Source: CAD feature listing. Evaluate the final solid. Frame: model axes, mm. A direction names the side the tool comes from. Give positions to 0.01 mm unless a question says otherwise; leave off trailing zeros. Write each loop counter-clockwise with the first axis right and the second up, starting at its lowest first coordinate (ties: lowest second). Pieces come first, ordered by that corner, then holes. Notation, with made-up numbers: (39, -34) -> (62, -34) arc R13 cw to (62, -10) -> close; hole circle Ø6 at (87, 86.5). An arc over 180 degrees is marked (long way). Write item = value, one per line.
from build123d import *

# Parameters (mm, degrees)
PAD_DEPTH   = 4
FILLET_R    = 25
SKETCH002_R = 1.25
HOLE_DEPTH  = 3
HOLE_TIPS_R = 1.25


with BuildPart() as part:
    # Sketch → Revolution (revolve)
    with BuildSketch(Plane.XZ):
        with BuildLine():
            Line((0, 0), (0, 17.5))
            Line((0, 17.5), (36, 20))
            Line((36, 20), (36, 21))
            Line((36, 21), (48, 21))
            Line((48, 21), (48, 17))
            Line((48, 17), (87, 21.424285))
            ThreePointArc((138, 0), (119.61895, 27.658633), (87, 21.424285))
            Line((138, 0), (0, 0))
        make_face()
    revolve(axis=Axis((0, 0, 0), (1, 0, 0)))

    # Sketch001 → Pad (new body, symmetric)
    with BuildSketch(Plane.XZ):
        Polygon((0, 0), (0, -30.625503), (21.543212, -32.51029), (21.412478, -34.004582), (-1.5, -32), (-1.5, 0), align=None)
    extrude(amount=PAD_DEPTH, both=True)

    # Fillet
    fillet_edges = [part.edges().sort_by_distance(p)[0] for p in [
        (87, 0, -21.424285),
    ]]
    fillet(fillet_edges, radius=FILLET_R)

    # Sketch002 (on Face15 of Fillet) → Hole (cut)
    with BuildSketch(Plane(origin=(-2.789765, 0, -31.88716), x_dir=(0.996195, 0, -0.087156), z_dir=(-0.087156, 0, -0.996195))):
        with Locations((8, 0)):
            Circle(SKETCH002_R)
        with Locations((21, 0)):
            Circle(SKETCH002_R)
    extrude(amount=-HOLE_DEPTH, mode=Mode.SUBTRACT)

    # Hole tips → Hole tip 1 section 0
    with BuildSketch(Plane(origin=(-2.528298, 0, -28.898576), x_dir=(0.996195, 0, -0.087156), z_dir=(-0.087156, 0, -0.996195)), mode=Mode.PRIVATE) as hole_tip_1_s0:
        with Locations((8, 0)):
            Circle(HOLE_TIPS_R)
    loft([hole_tip_1_s0.sketch, Vertex(5.50672, 0, -28.847604)], mode=Mode.SUBTRACT)

    # Hole tips → Hole tip 2 section 0
    with BuildSketch(Plane(origin=(-2.528298, 0, -28.898576), x_dir=(0.996195, 0, -0.087156), z_dir=(-0.087156, 0, -0.996195)), mode=Mode.PRIVATE) as hole_tip_2_s0:
        with Locations((21, 0)):
            Circle(HOLE_TIPS_R)
    loft([hole_tip_2_s0.sketch, Vertex(18.457251, 0, -29.980629)], mode=Mode.SUBTRACT)


solid = part.part
1) Material intervals for L1, parallel to Z at x = 84, y = -7; L2, parallel to Z at x = 95, y = -6; L3, parallel to Y at x = 69.5, z = -4, sorted ascending.
Computed:
L1 = -20.27 to 20.27
L2 = -26.36 to 26.36
L3 = -19.02 to 19.02
2) Access query for faces 4 (the flat face through (-0.2, 4, -22)), 5 (the flat face through (10.117, -0.056, -33.016)), 6 (the flat face through (10.621, -0.056, -31.555)), 7 (the flat face through (48, 15.5, 7.7)). Directions: +Z, -Z, +X, -X, +Y, -Y. A direction counts if a zero-diameter tool reaches every point of the face in a straight line with its end or side. Return the directions, or none.
Computed:
face_4 = -Z, -X, +Y
face_5 = -Z, -X, +Y, -Y
face_6 = +X, +Y, -Y
face_7 = none
3) Cut plane A-A (x = 28). Return the cut outline in (y, z), then the cut area to 3 significant figures.
Computed:
outline = circle Ø38.89 at (0, 0)
area = 1,190 mm²
4) Contact query for flat-ended pins moving along their axis: pin 1 (12 mm diameter, centred on y = 14.5, z = 6, fed in from -X); pin 2 (6 mm diameter, centred on x = 94.5, y = -16, fed in from +Z); pin 3 (10 mm diameter, centred on x = 89.5, y = -5, fed in from -Z); pin 4 (21 mm diameter, centred on y = 5, z = -2.5, fed in from +X). Output: stop coordinate, or through.
Computed:
pin_1 = 0
pin_2 = 24.05
pin_3 = -26.45
pin_4 = 138
5) Draft query along X for faces 1 (the flat face through (-1.5, 0, -16)), 2 (the cylindrical face through (6.43, -0.38, -31.95)), 3 (the flat face through (-0.2, -4, -22)). Return one class per face: pulls with the +X half, pulls with the -X half, needs draft (parallel to the pull), parting line crosses it, or undercut.
Computed:
face_1 = pulls with the -X half
face_2 = undercut
face_3 = needs draft
